Check sheet for the drawn part. Datum: minimum x, y, z corner. Units: mm. A direction names the side the tool comes from. Give positions to 0.01 mm unless a question says otherwise; leave off trailing zeros. Write each loop counter-clockwise with the first axis right and the second up, starting at its lowest first coordinate (ties: lowest second). Pieces come first, ordered by that corner, then holes. Notation, with made-up numbers: M -30,83.25 L -9,83.25 A21 cw -9,109.25 Z; hole C 77,-30 d5. An arc over 180 degrees is marked long. Write item = value, one per line.
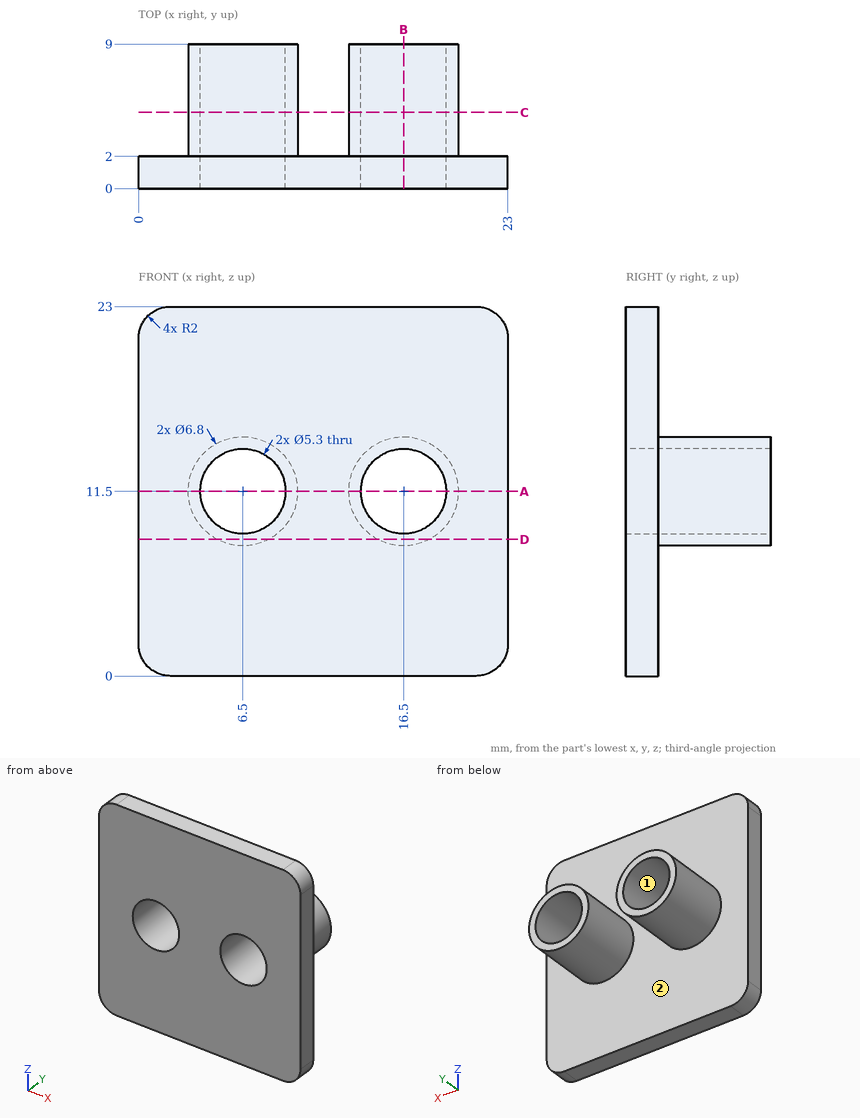
1) Depth check by flat-ended pin: P1, Ø4, axis at x = 10.5, y = 6.5, coming from the -Z side; P2, Ø1.5, axis at y = 4, z = 12.5, coming from the +X side. Enter the tip coordinate at first touch or a pass-through.
From the geometry:
P1 = 8.75
P2 = 19.89
2) Material ranges on probe 1 along X at (y, z) = (4.5, 11.5); probe 2 along Y at (x, z) = (10.5, 9.25); probe 3 along Z at (x, y) = (18.5, 4.5), recorded low to high. Write a range as from..to.
From the geometry:
probe_1 = 3.1..3.85, 9.15..9.9, 13.1..13.85, 19.15..19.9
probe_2 = 0..2
probe_3 = 8.75..9.76, 13.24..14.25
3) Cross-section at C-C on y = 4.75. Record the boundary of the cut face in (x, z), plus the area to 3 significant figures.
From the geometry:
outline = C 6.5,11.5 d6.8; C 16.5,11.5 d6.8; hole C 6.5,11.5 d5.3; hole C 16.5,11.5 d5.3
area = 28.5 mm^2
4) Tool access check on the marked faces 1 and 2. Record the directions out of +Z, -Z, +X, -X, +Y, -Y that give a thin tool (end or side, any length) a straight path to the whole face; none if there is none.
From the geometry:
face_1 = +Y, -Y
face_2 = +Y
5) Cross-section at A-A on z = 11.5. Record the boundary of the cut face in (x, y).
From the geometry:
outline = M 0,0 L 3.85,0 L 3.85,9 L 3.1,9 L 3.1,2 L 0,2 Z; M 9.15,0 L 13.85,0 L 13.85,9 L 13.1,9 L 13.1,2 L 9.9,2 L 9.9,9 L 9.15,9 Z; M 19.15,0 L 23,0 L 23,2 L 19.9,2 L 19.9,9 L 19.15,9 Z
6) Cross-section at B-B on x = 16.5. Record the boundary of the cut face in (y, z).
From the geometry:
outline = M 0,0 L 2,0 L 2,8.1 L 9,8.1 L 9,8.85 L 0,8.85 Z; M 0,14.15 L 9,14.15 L 9,14.9 L 2,14.9 L 2,23 L 0,23 Z
7) Cross-section at D-D on z = 8.5. Record the boundary of the cut face in (x, y), plus the area to 3 significant figures.
From the geometry:
outline = M 0,0 L 23,0 L 23,2 L 18.1,2 L 18.1,9 L 14.9,9 L 14.9,2 L 8.1,2 L 8.1,9 L 4.9,9 L 4.9,2 L 0,2 Z
area = 90.8 mm^2
